Part model, mm, in its own coordinate system. A direction names the side the tool comes from. Coordinates: 2 decimals unless noted, no trailing zeros. Loops run counter-clockwise (first coordinate to the right, second up) from the corner with the lowest first, then second, coordinate; pieces in that order, holes last. Notation, with made-up numbers: M -36.5,26 L 17.5,26 A15 cw 17.5,38 Z; hole C 20,8 d8. An arc over 180 degrees is marked long. Use a Markdown table: item, result. Add a question column.
1) Band-saw the part on B-B (z = -250). List the corners of the cut face in (x, y).
2) Band-saw the part on A-A (y = -5.5). List the corners of the cut face in (x, z), plus the area to 3 significant figures.
3) Wall check: probe 1 along X at (y, z) = (20.5, -122); probe 2 along Y at (x, z) = (6.5, 308); probe 3 along X at (y, z) = (-24.3, -88.9). Give the ranges that are in metal, low to high. Write a range as from..to.
4) Tool access for faces 4 (the flat face through (12.7, 0, -5)), 5 (the flat face through (-10.16, 0, -5)): list every direction of +Z, -Z, +X, -X, +Y, -Y with a clear straight run to the whole face (end or side of a thin tool).
5) Pin check, flat tip, straight feed: pin 1 Ø5 at (x, z) = (0, 139.7) entering from +Y. Stop position of the tip, or through.
6) Pull direction Y, two halves, no side cores. Call faces 1 (the flat face through (-12.7, 0, -5)), 2 (the flat face through (0, -25.4, -5)), 3 (the flat face through (0, -22.86, -5)): released by +Y, released by -Y, zero draft, split by the parting line, or undercut.
Autodesk Inventor part; units mm, degrees
ref_plane "YZ Plane" through (0, 0, 0) normal (1, 0, 0) x (0, 1, 0)
ref_plane "XZ Plane" through (0, 0, 0) normal (0, 1, 0) x (-1, 0, 0)
ref_plane "XY Plane" through (0, 0, 0) normal (0, 0, 1) x (1, 0, 0)
sketch "Sketch1" plane through (0, 0, 0) normal (0, 0, 1) x (1, 0, 0)
  line L0 (-12.7, -25.4) -> (12.7, -25.4)
  line L1 (12.7, -25.4) -> (12.7, 25.4)
  line L2 (12.7, 25.4) -> (-12.7, 25.4)
  line L3 (-12.7, 25.4) -> (-12.7, -25.4)
  line L4 (-12.7, -25.4) -> (12.7, 25.4) construction
  line L5 (12.7, -25.4) -> (-12.7, 25.4) construction
  line L6 (-10.16, -22.86) -> (10.16, -22.86)
  line L7 (10.16, -22.86) -> (10.16, 22.86)
  line L8 (10.16, 22.86) -> (-10.16, 22.86)
  line L9 (-10.16, 22.86) -> (-10.16, -22.86)
  line L10 (-10.16, -22.86) -> (10.16, 22.86) construction
  line L11 (10.16, -22.86) -> (-10.16, 22.86) construction
  point P0 (0, 0)
  dimension "d0" = 25.4
  dimension "d1" = 50.8
  dimension "d2" = 20.32
  dimension "d3" = 45.72
extrude "Extrusion1" add sketch "Sketch1" along normal mid plane 711.2
sketch "Sketch2" plane through (-12.7, 25.4, 355.6) normal (0, 1, 0) x (1, 0, 0)
  line L0 (25.4, 711.2) -> (25.4, 0)
  line L1 (25.4, 0) -> (0, 0)
  point P0 (12.7, 355.6)
  point P1 (12.7, 12.7)
  dimension "d6" = 12.7
  dimension "d7" = 12.7
hole "Hole1" at (0, 25.4, 342.9) direction (0, -1, 0) diameter 4.1402 end through all
pattern_linear "Rectangular Pattern1" count 28 spacing 25.4 along (0, 0, -1) of "Hole1"
properties part number "Drivetrain_width"
Entries:
| question | item | result |
|---|---|---|
| 1 | outline | M -12.7,-25.4 L 12.7,-25.4 L 12.7,25.4 L -12.7,25.4 Z; hole M -10.16,-22.86 L 10.16,-22.86 L 10.16,22.86 L -10.16,22.86 Z |
| 2 | outline | M -12.7,-355.6 L -10.16,-355.6 L -10.16,355.6 L -12.7,355.6 Z; M 10.16,-355.6 L 12.7,-355.6 L 12.7,355.6 L 10.16,355.6 Z |
| 2 | area | 3,610 mm2 |
| 3 | probe 1 | -12.7..-10.16, 10.16..12.7 |
| 3 | probe 2 | -25.4..-22.86, 22.86..25.4 |
| 3 | probe 3 | -12.7..-2.07, 2.07..12.7 |
| 4 | face 4 | +Z, -Z, +X, +Y, -Y |
| 4 | face 5 | +Z, -Z |
| 5 | pin 1 | y = 25.4 |
| 6 | face 1 | zero draft |
| 6 | face 2 | released by -Y |
| 6 | face 3 | undercut |
